The listing builds one solid part. Answer for the finished solid, in the listing's coordinates (mm). Face numbers are marked on the shaded views. A direction names the side the tool comes from. Coordinates: 2 decimals unless noted, no trailing zeros. Order: outer loops, then holes, each group sorted by start corner. A loop starts at its lowest first (then second) coordinate and runs counter-clockwise, first axis right, second up. Notation, with made-up numbers: (39, -36) - (77, -36) arc R11 cw to (77, -25) - close; hole circle Ø8 at (29.25, 80.25). An arc over 180 degrees is marked (long way). Use a Markdown table: item, result. Add a question column.
Item 1: The part is cut by section B-B, the plane x = 0. Give the vertices of the cut face in (y, z).
Item 2: The mould has two halves that part along X. Classify the marked faces 1, 2, 3 and 4: released by +X, released by -X, zero draft, split by the parting line, or undercut.
Item 3: The part is cut by section A-A, the plane x = 200. Give the vertices of the cut face in (y, z), then the cut area to 3 significant figures.
Item 4: For the marked faces 5, 6, 7 and 8, determine the directions among +Z, -Z, +X, -X, +Y, -Y from which every point of the face is accessible in a straight line to the end or side of a thin tool.
Item 5: The part is cut by section D-D, the plane z = 7.5. Give the vertices of the cut face in (x, y), then the cut area to 3 significant figures.
Item 6: Find the intervals of material crossed by line 1 along Z through (x, y) = (98.5, -2.5); line 2 along Z through (x, y) = (200, 6); line 3 along X through (y, z) = (-20, 16), in increasing order.
Item 7: The part is cut by section C-C, the plane y = 0. State how many separate pieces and enclosed holes the cut face has, then the cut area to 3 significant figures.
Item 8: Flat-ended cylindrical pins translate along their axes: P1, Ø8, axis at x = 181, z = 22, coming from the -Y side; P2, Ø1.5, axis at y = -0.5, z = 28, coming from the -X side; P3, Ø7.5, axis at x = 131, y = -2, coming from the +Z side. Find the tip coordinate at first contact, or state that the pin passes through.
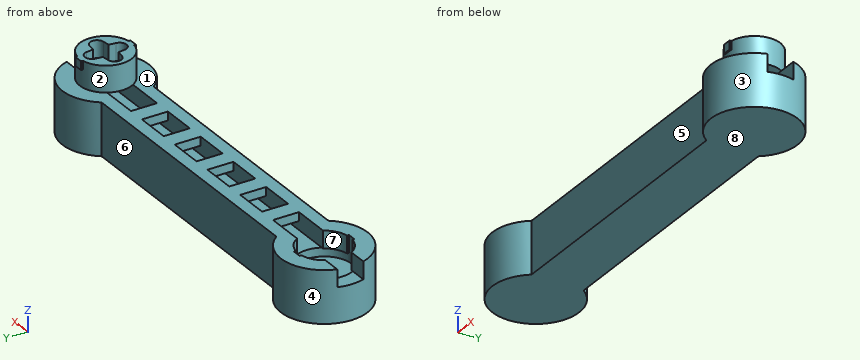
Autodesk Inventor part; units mm, degrees
ref_plane "YZ Plane" through (0, 0, 0) normal (1, 0, 0) x (0, 1, 0)
ref_plane "XZ Plane" through (0, 0, 0) normal (0, 1, 0) x (-1, 0, 0)
ref_plane "XY Plane" through (0, 0, 0) normal (0, 0, 1) x (1, 0, 0)
sketch "Szkic1" plane through (0, 0, 0) normal (0, 0, 1) x (1, 0, 0)
  arc A0 (20, 15) -> (-20, 15) centre (0, 0) ccw
  line L0 (20, 15) -> (100, 15)
  line L1 (100, 15) -> (100, -15)
  line L2 (100, -15) -> (20, -15)
  arc A1 (180, -15) -> (180, 15) centre (200, 0) ccw
  line L3 (180, 15) -> (100, 15)
  line L4 (100, -15) -> (180, -15)
  arc A2 (-20, 15) -> (20, -15) centre (0, 0) ccw
  dimension "d0" = 50
  dimension "d1" = 30
  dimension "d2" = 200
extrude "kształt" add sketch "Szkic1" along normal blind 30
sketch "Szkic2" plane through (0, 0, 30) normal (0, 0, 1) x (1, 0, 0)
  arc A0 (20, 15) -> (20, -15) centre (0, 0) ccw
  line L0 (20, -15) -> (180, -15)
  arc A1 (180, -15) -> (180, 15) centre (200, 0) ccw
  line L1 (180, 15) -> (20, 15)
  line L2 (-23.8485, 7.5) -> (223.8485, 7.5)
  line L3 (223.8485, -7.5) -> (-73.8485, -7.5)
  point P0 (-23.8485, -7.5)
  dimension "d5" = 15
extrude "rowek na kable" cut sketch "Szkic2" against normal blind 10 contours L2 A1 L3 A0
sketch "Szkic3" plane through (0, 0, 30) normal (0, 0, 1) x (1, 0, 0)
  arc A0 (223.8485, 7.5) -> (180, 15) centre (200, 0) ccw
  circle A1 centre (200, 0) radius 15
  point P0 (0, 0)
  dimension "d8" = 30
extrude "odstająćy cosik" add sketch "Szkic3" along normal blind 15
sketch "Szkic4" plane through (0, 0, 30) normal (0, 0, 1) x (1, 0, 0)
  circle A0 centre (0, 0) radius 15
  dimension "d11" = 30
extrude "wgłebiający cosik" cut sketch "Szkic4" against normal blind 15
sketch "Szkic5" plane through (0, 0, 30) normal (0, 0, 1) x (1, 0, 0)
  arc A0 (12.9904, 7.5) -> (-12.9904, 7.5) centre (0, 0) ccw
  line L0 (12.9904, 7.5) -> (187.0096, 7.5)
  arc A1 (212.9904, 7.5) -> (187.0096, 7.5) centre (200, 0) ccw
  line L1 (212.9904, 7.5) -> (223.8485, 7.5)
  arc A2 (223.8485, 7.5) -> (180, 15) centre (200, 0) ccw
  line L2 (180, 15) -> (20, 15)
  arc A3 (20, 15) -> (-23.8485, 7.5) centre (0, 0) ccw
  line L3 (-23.8485, 7.5) -> (-12.9904, 7.5)
  arc A4 (-12.9904, -7.5) -> (12.9904, -7.5) centre (0, 0) ccw
  line L4 (-12.9904, -7.5) -> (-23.8485, -7.5)
  arc A5 (-23.8485, -7.5) -> (20, -15) centre (0, 0) ccw
  line L5 (20, -15) -> (180, -15)
  arc A6 (180, -15) -> (223.8485, -7.5) centre (200, 0) ccw
  line L6 (223.8485, -7.5) -> (212.9904, -7.5)
  arc A7 (187.0096, -7.5) -> (212.9904, -7.5) centre (200, 0) ccw
  line L7 (187.0096, -7.5) -> (12.9904, -7.5)
  line L8 (35, 7.5) -> (45, 7.5)
  line L9 (45, 7.5) -> (45, -7.5)
  line L10 (45, -7.5) -> (35, -7.5)
  line L11 (35, -7.5) -> (35, 7.5)
  arc A8 (-23.8485, -7.5) -> (20, -15) centre (0, 0) ccw
  line L12 (65, -7.5) -> (65, 7.5)
  line L13 (75, 7.5) -> (75, -7.5)
  line L14 (75, -7.5) -> (65, -7.5)
  line L15 (65, 7.5) -> (75, 7.5)
  line L16 (95, -7.5) -> (95, 7.5)
  line L17 (105, 7.5) -> (105, -7.5)
  line L18 (105, -7.5) -> (95, -7.5)
  line L19 (95, 7.5) -> (105, 7.5)
  line L20 (125, -7.5) -> (125, 7.5)
  line L21 (135, 7.5) -> (135, -7.5)
  line L22 (135, -7.5) -> (125, -7.5)
  line L23 (125, 7.5) -> (135, 7.5)
  line L24 (155, -7.5) -> (155, 7.5)
  line L25 (165, 7.5) -> (165, -7.5)
  line L26 (165, -7.5) -> (155, -7.5)
  line L27 (155, 7.5) -> (165, 7.5)
  arc A9 (223.8485, 7.5) -> (180, 15) centre (200, 0) ccw
  line L28 (0, 0) -> (100, 0) construction
  line L29 (100, -7.5) -> (100, 7.5) construction
  line L30 (100, 0) -> (200, 0) construction
  point P0 (35, -7.5)
  point P1 (75, -7.5)
  point P2 (75, 7.5)
  point P3 (65, 7.5)
  point P4 (165, -7.5)
  point P5 (165, 7.5)
  point P6 (155, 7.5)
  point P7 (155, -7.5)
  point P8 (135, -7.5)
  point P9 (135, 7.5)
  point P10 (125, 7.5)
  point P11 (105, -7.5)
  point P12 (105, 7.5)
  point P13 (95, 7.5)
  dimension "d15" = 10
  dimension "d18" = 30
extrude "wzmocnienie" add sketch "Szkic5" against normal blind 5 contours L0 L9 L7 L11 | L0 L13 L7 L12 | L0 L17 L7 L16 | L0 L21 L7 L20 | L25 L7 L24 L0
sketch "Szkic6" plane through (200, 0, 45) normal (0, 0, 1) x (1, 0, 0)
  circle A0 centre (0, 0) radius 15
  arc A1 (2.5, 15.8035) -> (2.5, -15.8035) centre (0, 0) ccw construction
  line L0 (-2.5, 15.8035) -> (2.5, 15.8035)
  line L1 (2.5, 15.8035) -> (2.5, 14.7902)
  line L2 (2.5, -15.8035) -> (-2.5, -15.8035)
  line L3 (-2.5, -15.8035) -> (-2.5, -14.7902)
  line L4 (2.5, 14.7902) -> (2.5, -14.7902) construction
  line L5 (-2.5, 14.7902) -> (-2.5, 15.8035)
  line L6 (-2.5, -14.7902) -> (-2.5, 14.7902) construction
  line L7 (2.5, -14.7902) -> (2.5, -15.8035)
  point P0 (-200, 0)
  dimension "d25" = 32
  dimension "d27" = 5
extrude "złobek" add sketch "Szkic6" against normal blind 5 contours A0 L5 L0 L1 | L7 L2 L3 A0
sketch "Szkic7" plane through (0, 0, 30) normal (0, 0, 1) x (1, 0, 0)
  circle A0 centre (0, 0) radius 16 construction
  line L0 (-2.5, 15.8035) -> (2.5, 15.8035)
  line L1 (2.5, -15.8035) -> (-2.5, -15.8035)
  arc A1 (12.9904, 7.5) -> (-12.9904, 7.5) centre (0, 0) ccw
  arc A2 (-12.9904, -7.5) -> (12.9904, -7.5) centre (0, 0) ccw
  line L2 (2.5, 15.8035) -> (2.5, 14.7902)
  line L3 (2.5, -14.7902) -> (2.5, -15.8035)
  line L4 (-2.5, -15.8035) -> (-2.5, -14.7902)
  line L5 (-2.5, 14.7902) -> (-2.5, 15.8035)
  arc A3 (2.5, 14.7902) -> (-2.5, 14.7902) centre (0, 0) ccw
  arc A4 (-2.5, -14.7902) -> (2.5, -14.7902) centre (0, 0) ccw
  point P0 (2.5, 15.2968)
  dimension "d30" = 32
  dimension "d32" = 5
extrude "wklęsły żłobek" cut sketch "Szkic7" against normal up to surface (15 mm away)
sketch "Szkic8" plane through (0, 0, 15) normal (0, 0, 1) x (1, 0, 0)
  arc A0 (2.5, -14.7902) -> (2.5, 14.7902) centre (0, 0) ccw
  line L0 (2.5, 15.8035) -> (2.5, 14.7902)
  line L1 (-2.5, 15.8035) -> (2.5, 15.8035)
  line L2 (-2.5, 14.7902) -> (-2.5, 15.8035)
  arc A1 (-2.5, 14.7902) -> (-2.5, -14.7902) centre (0, 0) ccw
  line L3 (-2.5, -15.8035) -> (-2.5, -14.7902)
  line L4 (2.5, -15.8035) -> (-2.5, -15.8035)
  line L5 (2.5, -14.7902) -> (2.5, -15.8035)
  circle A2 centre (0, 0) radius 16
  circle A3 centre (0, 0) radius 15
extrude "rowek" cut sketch "Szkic8" along normal blind 5 contours A0 L0 A2 L5 | L3 A2 L2 A1
sketch "Szkic12" plane through (0, 0, 45) normal (0, 0, 1) x (1, 0, 0)
  arc A0 (202.5, -14.7902) -> (202.5, 14.7902) centre (200, 0) ccw
  circle A1 centre (200, 0) radius 5 construction
  arc A2 (203.9686, 8.5) -> (196.0314, 8.5) centre (200, 8) ccw
  line L0 (195.0392, 0.625) -> (196.0314, 8.5)
  line L1 (204.9608, 0.625) -> (203.9686, 8.5)
  line L2 (199.375, 4.9608) -> (191.5, 3.9686)
  arc A3 (191.5, 3.9686) -> (191.5, -3.9686) centre (192, 0) ccw
  line L3 (199.375, -4.9608) -> (191.5, -3.9686)
  line L4 (195.0392, -0.625) -> (196.0314, -8.5)
  arc A4 (196.0314, -8.5) -> (203.9686, -8.5) centre (200, -8) ccw
  line L5 (204.9608, -0.625) -> (203.9686, -8.5)
  line L6 (200.625, -4.9608) -> (208.5, -3.9686)
  arc A5 (208.5, -3.9686) -> (208.5, 3.9686) centre (208, 0) ccw
  line L7 (200.625, 4.9608) -> (208.5, 3.9686)
  point P0 (0, 0)
  point P1 (195.5244, 4.4756)
  point P2 (195.5244, -4.4756)
  point P3 (204.4756, -4.4756)
  point P4 (204.4756, 4.4756)
  dimension "d53" = 10
  dimension "d54" = 8
  dimension "d55" = 8
  dimension "d58" = 360
extrude "Wyciągnięcie proste12" cut sketch "Szkic12" against normal blind 10
properties part number "2stopien" material "Tworzywo sztuczne ABS"
Solution:
| question | item | result |
|---|---|---|
| 1 | outline | (-25, 0) - (25, 0) - (25, 30) - (15.8, 30) - (15.8, 15) - (-15.8, 15) - (-15.8, 30) - (-25, 30) - close |
| 2 | face 1 | zero draft |
| 2 | face 2 | split by the parting line |
| 2 | face 3 | undercut |
| 2 | face 4 | undercut |
| 3 | outline | (-25, 0) - (25, 0) - (25, 30) - (15, 30) - (15, 40) - (15.8, 40) - (15.8, 45) - (12, 45) - (12, 35) - (-12, 35) - (-12, 45) - (-15.8, 45) - (-15.8, 40) - (-15, 40) - (-15, 30) - (-25, 30) - close; hole (-7.5, 20) - (7.5, 20) - (7.5, 30) - (-7.5, 30) - close |
| 3 | area | 1,570 mm2 |
| 4 | face 5 | +Z, -Z, -Y |
| 4 | face 6 | +Z, -Z, +Y |
| 4 | face 7 | +Z |
| 4 | face 8 | -Z, +X, -X, +Y, -Y |
| 5 | outline | (20, -15) - (180, -15) arc R25 ccw (long way) to (180, 15) - (20, 15) arc R25 ccw (long way) to start |
| 5 | area | 8,520 mm2 |
| 6 | line 1 | z = 0 to 20, 25 to 30 |
| 6 | line 2 | z = 0 to 20, 30 to 35 |
| 6 | line 3 | x = -15 to 15, 185 to 215 |
| 7 | separate pieces | 7 |
| 7 | enclosed holes | 0 |
| 7 | area | 5,300 mm2 |
| 8 | P1 | stops at y = -20 |
| 8 | P2 | stops at x = 35 |
| 8 | P3 | stops at z = 30 |
